Input: part model. Units: mm. Frame: model coordinates. A direction names the side the tool comes from. Give positions to 0.01 mm unless a question says otherwise; leave off trailing zeros. Write each loop counter-clockwise with the first axis right and the second up, starting at its lowest first coordinate (ties: lowest second). Pieces come first, ordered by that corner, then holes. Notation, with made-up numbers: (45.25, 10.5) - (88.25, 10.5) arc R26 cw to (88.25, 47.5) - close; hole circle Ø10 at (20.25, 87.5). An arc over 180 degrees is marked (long way). Answer as CSV lines item,"result".
```python
from build123d import *

# Parameters (mm, degrees)
BOSS_EXTRUDE1_DEPTH                  = 3
SKETCH10_W                           = 17.5
SKETCH10_H                           = 24
BOSS_EXTRUDE2_DEPTH                  = 3
F_2_5_2_5_DIAMETER_HOLE1_D           = 2.5
F_2_5_2_5_DIAMETER_HOLE1_DEPTH       = 6.35
F_2_5_2_5_DIAMETER_HOLE1_CSINK_D     = 2.55
F_2_5_2_5_DIAMETER_HOLE1_CSINK_ANGLE = 90
F_2_5_2_5_DIAMETER_HOLE1_TIP         = 0.751075774
M5X0_8_TAPPED_HOLE1_D                = 4.2
M5X0_8_TAPPED_HOLE1_DEPTH            = 12.4
M5X0_8_TAPPED_HOLE1_CSINK_D          = 5.05
M5X0_8_TAPPED_HOLE1_CSINK_ANGLE      = 90
M5X0_8_TAPPED_HOLE1_TIP              = 1.2618073
CUT_EXTRUDE3_DEPTH                   = 4
FILLET1_R                            = 3


with BuildPart() as part:
    # Sketch2 → Boss-Extrude1 (new body)
    with BuildSketch(Plane(origin=(0, 0, 0), x_dir=(1, 0, 0), z_dir=(0, 1, 0))):
        Polygon((42.5, 0), (42.5, 50), (22.5, 50), (8.75, 26.184301396), (-8.75, 26.184301396), (-22.5, 50), (-42.5, 50), (-42.5, 0), align=None)
    extrude(amount=BOSS_EXTRUDE1_DEPTH)

    # Sketch10 → Boss-Extrude2 (add)
    with BuildSketch(Plane(origin=(0, 3, 0), x_dir=(1, 0, 0), z_dir=(0, 1, 0))):
        with Locations((0, -12)):
            Rectangle(SKETCH10_W, SKETCH10_H)
    extrude(amount=-BOSS_EXTRUDE2_DEPTH)

    # Ø2.5 (2.5) Diameter Hole1
    with Locations(Plane(origin=(0, 3, 0), x_dir=(1, 0, 0), z_dir=(0, 1, 0))):
        with Locations((0, -19), (0, -6)):
            CounterSinkHole(F_2_5_2_5_DIAMETER_HOLE1_D / 2, F_2_5_2_5_DIAMETER_HOLE1_CSINK_D / 2, depth=F_2_5_2_5_DIAMETER_HOLE1_DEPTH, counter_sink_angle=F_2_5_2_5_DIAMETER_HOLE1_CSINK_ANGLE)
            with Locations((0, 0, -(F_2_5_2_5_DIAMETER_HOLE1_DEPTH + F_2_5_2_5_DIAMETER_HOLE1_TIP / 2))):  # 118° drill point
                Cone(0, F_2_5_2_5_DIAMETER_HOLE1_D / 2, F_2_5_2_5_DIAMETER_HOLE1_TIP, mode=Mode.SUBTRACT)

    # M5x0.8 Tapped Hole1
    with Locations(Plane(origin=(0, 3, 0), x_dir=(1, 0, 0), z_dir=(0, 1, 0))):
        with Locations((-36.5, 40), (36.5, 40), (-36.5, 10), (36.5, 10)):
            CounterSinkHole(M5X0_8_TAPPED_HOLE1_D / 2, M5X0_8_TAPPED_HOLE1_CSINK_D / 2, depth=M5X0_8_TAPPED_HOLE1_DEPTH, counter_sink_angle=M5X0_8_TAPPED_HOLE1_CSINK_ANGLE)
            with Locations((0, 0, -(M5X0_8_TAPPED_HOLE1_DEPTH + M5X0_8_TAPPED_HOLE1_TIP / 2))):  # 118° drill point
                Cone(0, M5X0_8_TAPPED_HOLE1_D / 2, M5X0_8_TAPPED_HOLE1_TIP, mode=Mode.SUBTRACT)

    # Sketch9 → Cut-Extrude3 (cut, through all)
    with BuildSketch(Plane.XZ):
        Polygon((-32, -50), (-25, -26.184301396), (25, -26.184301396), (32, -50), align=None)
    extrude(amount=-CUT_EXTRUDE3_DEPTH, mode=Mode.SUBTRACT)

    # Fillet1
    fillet1_edges = [part.edges().sort_by_distance(p)[0] for p in [
        (25, 1.5, -26.184301396),
        (-42.5, 1.5, 0),
        (-42.5, 1.5, -50),
        (42.5, 1.5, -50),
        (42.5, 1.5, 0),
        (-8.75, 1.5, 0),
        (8.75, 1.5, 0),
        (32, 1.5, -50),
        (-25, 1.5, -26.184301396),
        (-32, 1.5, -50),
    ]]
    fillet(fillet1_edges, radius=FILLET1_R)


solid = part.part
```
Item 1: Cut plane D-D on y = 0.7. Return the cut outline in (x, z), plus the area to 3 significant figures.
The answers:
outline,"(-42.5, -47) arc R3 ccw to (-39.5, -50) - (-34.25, -50) arc R3 ccw to (-31.37, -47.85) - (-25.63, -28.34) arc R3 cw to (-22.75, -26.18) - (22.75, -26.18) arc R3 cw to (25.63, -28.34) - (31.37, -47.85) arc R3 ccw to (34.25, -50) - (39.5, -50) arc R3 ccw to (42.5, -47) - (42.5, -3) arc R3 ccw to (39.5, 0) - (11.75, 0) arc R3 cw to (8.75, 3) - (8.75, 24) - (-8.75, 24) - (-8.75, 3) arc R3 cw to (-11.75, 0) - (-39.5, 0) arc R3 ccw to (-42.5, -3) - close; hole circle Ø4.2 at (-36.5, -40); hole circle Ø4.2 at (-36.5, -10); hole circle Ø2.5 at (0, 6); hole circle Ø2.5 at (0, 19); hole circle Ø4.2 at (36.5, -40); hole circle Ø4.2 at (36.5, -10)"
area,"3,240 mm²"
Item 2: Reachability of faces 4 (the face through (8.75, 2, 14)), 5 (the face through (-8.75, 2, 14)), 6 (the face through (24.531, 1.521, -26.766)) from +Z, -Z, +X, -X, +Y, -Y: full face, straight path, thin tool, end or side. Return the list, or none.
The answers:
face 4,"+Z, +X, +Y, -Y"
face 5,"+Z, -X, +Y, -Y"
face 6,"-Z, +Y, -Y"
Item 3: Contact query for flat-ended pins moving along their axis: pin 1 (1.5 mm diameter, centred on y = 1.5, z = 13, fed in from +X); pin 2 (1.5 mm diameter, centred on x = -1.5, y = 2, fed in from -Z); pin 3 (0.9 mm diameter, centred on y = 1, z = 10.5, fed in from -X). Output: stop coordinate, or through.
The answers:
pin 1,"x = 8.75"
pin 2,"z = -26.18"
pin 3,"x = -8.75"
Item 4: Ray query, line 1 (Z direction, x = 0, y = 1.3); line 2 (X direction, y = 0.7, z = 19); line 3 (X direction, y = 2.3, z = -41). Return the intervals inside material, ascending. Write a range as from..to.
The answers:
line 1,"-26.18..4.75, 7.25..17.75, 20.25..24"
line 2,"-8.75..-1.25, 1.25..8.75"
line 3,"-42.5..-38.35, -34.65..-29.35, 29.35..34.65, 38.35..42.5"
Item 5: Cut plane B-B on x = 0. Return the cut outline in (y, z) (3 decimals), plus the area to 3 significant figures.
The answers:
outline,"(0, -26.184) - (3, -26.184) - (3, 4.725) - (2.975, 4.75) - (0, 4.75) - close; (0, 7.25) - (2.975, 7.25) - (3, 7.275) - (3, 17.725) - (2.975, 17.75) - (0, 17.75) - close; (0, 20.25) - (2.975, 20.25) - (3, 20.275) - (3, 24) - (0, 24) - close"
area,"136 mm²"
Item 6: Cut plane C-C on z = -10. Return the cut outline in (x, y) (3 decimals).
The answers:
outline,"(-42.5, 0) - (-38.6, 0) - (-38.6, 2.575) - (-39.025, 3) - (-42.5, 3) - close; (-34.4, 0) - (34.4, 0) - (34.4, 2.575) - (33.975, 3) - (-33.975, 3) - (-34.4, 2.575) - close; (38.6, 0) - (42.5, 0) - (42.5, 3) - (39.025, 3) - (38.6, 2.575) - close"
Item 7: Mould query, pull axis Z, two halves, no side actions, for faces 1 (the face through (0.27, 1.47, 20.22)), 2 (the face through (42.5, 1, -25)), 3 (the face through (32.43, 1.52, -49.39)). Classes: +Z half, -Z half, draft (parallel to the pull), parting line (faces both ways), or undercut.
The answers:
face 1,"undercut"
face 2,"draft"
face 3,"-Z half"
Item 8: Cut plane A-A on z = 6. Return the cut outline in (x, y) (3 decimals), plus the area to 3 significant figures.
The answers:
outline,"(-8.75, 0) - (-1.25, 0) - (-1.25, 2.975) - (-1.275, 3) - (-8.75, 3) - close; (1.25, 0) - (8.75, 0) - (8.75, 3) - (1.275, 3) - (1.25, 2.975) - close"
area,"45.0 mm²"
